Model file for the job. Use its own axes, mm. A direction names the side the tool comes from. Round coordinates to 2 decimals unless told otherwise and drop trailing zeros. Order: outer loops, then holes, each group sorted by start corner. A loop starts at its lowest first (then second) coordinate and runs counter-clockwise, first axis right, second up. Notation, with made-up numbers: (62.5, 2.5) - (86.5, 2.5) arc R22 cw to (86.5, 26.5) - close; hole circle Ø7 at (-37, 13.5). An arc over 180 degrees is marked (long way). Use one line per item in the form item = value.
Autodesk Inventor part; units mm, degrees
ref_plane "YZ Plane" through (0, 0, 0) normal (1, 0, 0) x (0, 1, 0)
ref_plane "XZ Plane" through (0, 0, 0) normal (0, 1, 0) x (-1, 0, 0)
ref_plane "XY Plane" through (0, 0, 0) normal (0, 0, 1) x (1, 0, 0)
sketch "Sketch1" plane through (0, 0, 0) normal (1, 0, 0) x (0, 1, 0)
  line L0 (-191.1, 0) -> (191.1, 0) construction
  line L1 (0, -45.54) -> (0, 63.24) construction
  line L2 (-136.5, 30) -> (136.5, 30)
  line L3 (136.5, 30) -> (136.5, -30)
  line L4 (136.5, -30) -> (-136.5, -30)
  line L5 (-136.5, -30) -> (-136.5, 30)
  line L6 (109.0139, 30) -> (136.5, 47.7)
  line L7 (136.5, 47.7) -> (136.5, 30)
  circle A0 centre (133.5, 42.1999) radius 3
  circle A1 centre (115.5, 30.6086) radius 3
  line L8 (-136.5, 30) -> (103.5, 30) construction
  line L9 (103.5, 30) -> (103.5, 38) construction
  line L10 (103.5, 38) -> (-136.5, 38) construction
  line L11 (-136.5, 38) -> (-136.5, 30) construction
  line L12 (112.5, 32.2449) -> (112.5, 30)
  circle A2 centre (109.5, 30) radius 3
  circle A3 centre (109.5, 33) radius 3
  line L13 (-56.5, 30) -> (3.5, 30)
  line L14 (3.5, 30) -> (3.5, 6.4132)
  line L15 (3.5, 6.4132) -> (-56.5, 6.4132)
  line L16 (-56.5, 6.4132) -> (-56.5, 30)
  line L17 (-26.5, 6.4132) -> (-26.5, 30) construction
  point P0 (0, 0)
  point P1 (106.5, 30)
  dimension "d6" = 6
  dimension "d1" = 32.78
  dimension "d2" = 6
  dimension "d3" = 8
  dimension "d4" = 240
  dimension "d7" = 60
  dimension "d35" = 147.22
  dimension "d36" = 273
  dimension "d37" = 17.7
  dimension "d38" = 24
  dimension "d39" = 110
  dimension "d40" = 60
extrude "Extrusion1" add sketch "Sketch1" along normal mid plane 10 contours L2 L16 L15 L14 A2 A1 L3 L4 L5 | L2 L14 L15 L16 | L2 A2 | L2 A1 L6 A0 L7 | L6 A3 L2 | L12 A1 L2 | A2 A3 L6 L12 | L2 A3 A2 | A1 L2 | L2 A1 | A0 L6 L7 | A0 | A3 L6 A2 | L6 A3 A2 | L12 L6 A1 picked at (110.4979, 30.6349) picked at (112.1863, 31.9825)
sketch "Sketch2" plane through (-5, -136.5, 30) normal (0, 0, 1) x (1, 0, 0)
  line L0 (5, -54.6) -> (5, 327.6) construction
  line L1 (0, 0) -> (10, 0)
  point P0 (5, 136.5)
  point P1 (5, 72.5)
  point P2 (5, 147.5)
  point P3 (5, 222.5)
  dimension "d11" = 72.5
  dimension "d12" = 75
  dimension "d13" = 75
hole "Hole1" at (0, -64, 30) at (0, 11, 30) at (0, 86, 30) direction (0, 0, -1) diameter 3.242 depth 15 tip angle 118
sketch "Sketch3" plane through (5, 136.5, -30) normal (0, 0, -1) x (-1, 0, 0)
  line L0 (12, -136.5) -> (-2, -136.5) construction
  line L1 (5, -327.6) -> (5, 54.6) construction
  point P0 (5, -136.5)
  point P1 (5, -261.5)
  point P2 (5, -136.5)
  point P3 (5, -11.5)
  dimension "d21" = 250
hole "Hole2" at (0, -125, -30) at (0, 0, -30) at (0, 125, -30) direction (0, 0, 1) diameter 3.242 depth 15 tip angle 118
fillet "Fillet1" radius 3 2 edges at (0, 136.5, 47.7) (0, 109.0139, 30)
chamfer "Chamfer1" distance 1 angle 45 1 edges at (0, -136.5, 30)
properties part number "GRJ-04-102" material "Fenolite OR"
(1) Tool access for faces 1 (the face through (-5, -2, 0)), 2 (the face through (0, -15, 30)): list every direction of +Z, -Z, +X, -X, +Y, -Y with a clear straight run to the whole face (end or side of a thin tool).
Report:
face_1 = +Z, -Z, -X, +Y, -Y
face_2 = +Z, +X, -X, -Y
(2) Pin check, flat tips, straight feed: pin 1 (3 mm diameter, centred on x = -1, y = -48.5, fed in from +Z); pin 2 (1.9 mm diameter, centred on x = 0, y = 0, fed in from -Z). Stop position of each tip, or through.
Report:
pin_1 = 30
pin_2 = -14.6
(3) Slice it at C-C on z = 37. Give the cut face in (x, y), then the cut area to 3 significant figures.
Report:
outline = (-5, 119.88) - (5, 119.88) - (5, 136.5) - (-5, 136.5) - close
area = 166 mm2
(4) Probe probe 1 along Y at (x, z) = (0, 20.25); probe 2 along X at (y, z) = (-64, 25); probe 3 along Z at (x, y) = (4.25, 37.5). List the from-to ranges inside material, lowest first. Write a range as [from, to].
Report:
probe_1 = [-136.5, -65.62], [-62.38, 9.38], [12.62, 84.38], [87.62, 136.5]
probe_2 = [-5, -1.62], [1.62, 5]
probe_3 = [-30, 30]
(5) Slice it at A-A on x = 3.5. Give the cut face in (y, z), then the cut area to 3 significant figures.
Report:
outline = (-136.5, -30) - (136.5, -30) - (136.5, 42.2) arc R3 ccw to (131.88, 44.72) - (109.76, 30.48) arc R3 cw to (108.13, 30) - (-135.5, 30) - (-136.5, 29) - close
area = 16,600 mm2
(6) Slice it at B-B on y = -76. Give the cut face in (x, z).
Report:
outline = (-5, -30) - (5, -30) - (5, 30) - (-5, 30) - close
